Work out the finished part from the listing and answer in its coordinate system (mm). Coordinates: 2 decimals unless noted, no trailing zeros. Order: outer loops, then holes, each group sorted by start corner. A loop starts at its lowest first (then second) coordinate and runs counter-clockwise, first axis right, second up.
1. The part is cut by section B-B, the plane y = 0. Give the vertices of the cut face in (x, z), then the cut area to 3 significant figures.
2. Find the intervals of material crossed by probe 1 along Y at (x, z) = (-32, 6.3); probe 2 along Y at (x, z) = (-45.5, 7.5); probe 3 along X at (y, z) = (14, 6.5), in increasing order.
3. The part is cut by section A-A, the plane y = -39. Give the vertices of the cut face in (x, z).
4. Flat-ended cylindrical pins translate along their axes: pin 1 Ø3 at (x, y) = (-32, -39) entering from +Z; pin 2 Ø1.1 at (x, z) = (-32, 4) entering from +Y. Find the tip coordinate at first contact, or state that the pin passes through.
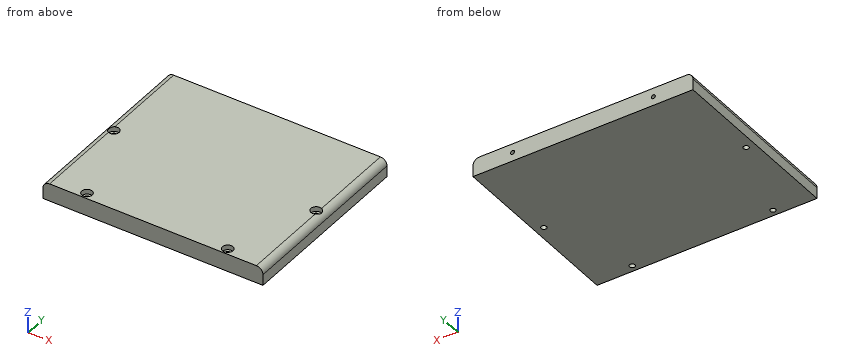
```python
from build123d import *

# Parameters (mm, degrees)
SKETCH1_W                                      = 100
SKETCH1_H                                      = 84
BOSS_EXTRUDE1_DEPTH                            = 8
CBORE_FOR_2_SOCKET_HEAD_CAP_SCREW1_D           = 2.4384
CBORE_FOR_2_SOCKET_HEAD_CAP_SCREW1_DEPTH       = 12.27
CBORE_FOR_2_SOCKET_HEAD_CAP_SCREW1_CBORE_D     = 4.7625
CBORE_FOR_2_SOCKET_HEAD_CAP_SCREW1_CBORE_DEPTH = 2.1844
CBORE_FOR_2_SOCKET_HEAD_CAP_SCREW1_TIP         = 0.732569267
CBORE_FOR_2_SOCKET_HEAD_CAP_SCREW2_D           = 2.4384
CBORE_FOR_2_SOCKET_HEAD_CAP_SCREW2_DEPTH       = 12.27
CBORE_FOR_2_SOCKET_HEAD_CAP_SCREW2_CBORE_D     = 4.7625
CBORE_FOR_2_SOCKET_HEAD_CAP_SCREW2_CBORE_DEPTH = 2.1844
CBORE_FOR_2_SOCKET_HEAD_CAP_SCREW2_TIP         = 0.732569267
F_2_56_TAPPED_HOLE1_D                          = 1.778
F_2_56_TAPPED_HOLE1_DEPTH                      = 12
F_2_56_TAPPED_HOLE1_TIP                        = 0.53416509
FILLET1_R                                      = 3


with BuildPart() as part:
    # Sketch1 → Boss-Extrude1 (new body)
    with BuildSketch(Plane.XY):
        Rectangle(SKETCH1_W, SKETCH1_H)
    extrude(amount=BOSS_EXTRUDE1_DEPTH)

    # CBORE for #2 Socket Head Cap Screw1
    with Locations(Plane(origin=(-32, -39, 8), x_dir=(1, 0, 0), z_dir=(0, 0, 1))):
        with Locations((0, 0), (64, 0)):
            CounterBoreHole(CBORE_FOR_2_SOCKET_HEAD_CAP_SCREW1_D / 2, CBORE_FOR_2_SOCKET_HEAD_CAP_SCREW1_CBORE_D / 2, CBORE_FOR_2_SOCKET_HEAD_CAP_SCREW1_CBORE_DEPTH, depth=CBORE_FOR_2_SOCKET_HEAD_CAP_SCREW1_DEPTH)
            with Locations((0, 0, -(CBORE_FOR_2_SOCKET_HEAD_CAP_SCREW1_DEPTH + CBORE_FOR_2_SOCKET_HEAD_CAP_SCREW1_TIP / 2))):  # 118° drill point
                Cone(0, CBORE_FOR_2_SOCKET_HEAD_CAP_SCREW1_D / 2, CBORE_FOR_2_SOCKET_HEAD_CAP_SCREW1_TIP, mode=Mode.SUBTRACT)

    # CBORE for #2 Socket Head Cap Screw2
    with Locations(Plane(origin=(-46, 0, 8), x_dir=(1, 0, 0), z_dir=(0, 0, 1))):
        with Locations((0, 0), (92, 0)):
            CounterBoreHole(CBORE_FOR_2_SOCKET_HEAD_CAP_SCREW2_D / 2, CBORE_FOR_2_SOCKET_HEAD_CAP_SCREW2_CBORE_D / 2, CBORE_FOR_2_SOCKET_HEAD_CAP_SCREW2_CBORE_DEPTH, depth=CBORE_FOR_2_SOCKET_HEAD_CAP_SCREW2_DEPTH)
            with Locations((0, 0, -(CBORE_FOR_2_SOCKET_HEAD_CAP_SCREW2_DEPTH + CBORE_FOR_2_SOCKET_HEAD_CAP_SCREW2_TIP / 2))):  # 118° drill point
                Cone(0, CBORE_FOR_2_SOCKET_HEAD_CAP_SCREW2_D / 2, CBORE_FOR_2_SOCKET_HEAD_CAP_SCREW2_TIP, mode=Mode.SUBTRACT)

    # #2-56 Tapped Hole1
    with Locations(Plane(origin=(-32, 42, 4), x_dir=(0, 0, 1), z_dir=(0, 1, 0))):
        with Locations((0, 0), (0, 64)):
            Hole(F_2_56_TAPPED_HOLE1_D / 2, depth=F_2_56_TAPPED_HOLE1_DEPTH)
            with Locations((0, 0, -(F_2_56_TAPPED_HOLE1_DEPTH + F_2_56_TAPPED_HOLE1_TIP / 2))):  # 118° drill point
                Cone(0, F_2_56_TAPPED_HOLE1_D / 2, F_2_56_TAPPED_HOLE1_TIP, mode=Mode.SUBTRACT)

    # Fillet1
    # the kernel refuses this fillet: 3 mm, written as the material it takes off along each edge
    with BuildSketch(Plane(origin=(-50, -49.5, 8), x_dir=(0, 0, -1), z_dir=(0, 1, 0))) as fillet1_piece_1:
        with BuildLine():
            CenterArc((FILLET1_R, -FILLET1_R), FILLET1_R, 90, 90)
            Line((0, -FILLET1_R), (0, 0))
            Line((0, 0), (FILLET1_R, 0))
        make_face()
    extrude(amount=99, mode=Mode.SUBTRACT)
    with BuildSketch(Plane(origin=(50, 49.5, 8), x_dir=(-1, 0, 0), z_dir=(0, -1, 0))) as fillet1_piece_2:
        with BuildLine():
            CenterArc((FILLET1_R, FILLET1_R), FILLET1_R, 180, 90)
            Line((0, FILLET1_R), (0, 0))
            Line((0, 0), (FILLET1_R, 0))
        make_face()
    extrude(amount=99, mode=Mode.SUBTRACT)


solid = part.part
```
Geometry says:
1. outline: (-50, 0) - (-47.22, 0) - (-47.22, 5.82) - (-48.38, 5.82) - (-48.38, 7.66) arc R3 ccw to (-50, 5) - close; (-44.78, 0) - (44.78, 0) - (44.78, 5.82) - (43.62, 5.82) - (43.62, 8) - (-43.62, 8) - (-43.62, 5.82) - (-44.78, 5.82) - close; (47.22, 0) - (50, 0) - (50, 5) arc R3 ccw to (48.38, 7.66) - (48.38, 5.82) - (47.22, 5.82) - close
1. area: 747 mm2
2. probe 1: y = -42 to -41.38, -36.62 to 42
2. probe 2: y = -42 to -2.33, 2.33 to 42
2. probe 3: x = -49.6 to 49.6
3. outline: (-50, 0) - (-33.22, 0) - (-33.22, 5.82) - (-34.38, 5.82) - (-34.38, 8) - (-47, 8) arc R3 ccw to (-50, 5) - close; (-30.78, 0) - (30.78, 0) - (30.78, 5.82) - (29.62, 5.82) - (29.62, 8) - (-29.62, 8) - (-29.62, 5.82) - (-30.78, 5.82) - close; (33.22, 0) - (50, 0) - (50, 5) arc R3 ccw to (47, 8) - (34.38, 8) - (34.38, 5.82) - (33.22, 5.82) - close
4. pin 1: stops at z = 5.82
4. pin 2: stops at y = 29.8
